```python
from build123d import *

# Parameters (mm, degrees)
BOSS_EXTRUDE1_DEPTH = 10
SKETCH2_R           = 11.75
BOSS_EXTRUDE2_DEPTH = 40
BOSS_EXTRUDE3_DEPTH = 20
CUT_EXTRUDE1_DEPTH  = 16
CUT_EXTRUDE2_DEPTH  = 10
CHAMFER1_SIZE       = 2
CHAMFER1_SIZE2      = 5.494954839


with BuildPart() as part:
    # Sketch1 → Boss-Extrude1 (new body)
    with BuildSketch(Plane(origin=(0, 0, 0), x_dir=(1, 0, 0), z_dir=(0, 1, 0))):
        Polygon((21.75, 12.557368355), (0, 25.11473671), (-21.75, 12.557368355), (-21.75, -12.557368355), (0, -25.11473671), (21.75, -12.557368355), align=None)
        Polygon((15.25, 8.804591605), (0, 17.60918321), (-15.25, 8.804591605), (-15.25, -8.804591605), (0, -17.60918321), (15.25, -8.804591605), align=None, mode=Mode.SUBTRACT)
    extrude(amount=BOSS_EXTRUDE1_DEPTH)

    # Sketch2 → Boss-Extrude2 (add)
    with BuildSketch(Plane.XZ):
        Polygon((21.75, 12.557368355), (0, 25.11473671), (-21.75, 12.557368355), (-21.75, -12.557368355), (0, -25.11473671), (21.75, -12.557368355), align=None)
        with Locations(Location((0, 0, 0), (0, 0, 270))):
            Circle(SKETCH2_R, mode=Mode.SUBTRACT)
    extrude(amount=BOSS_EXTRUDE2_DEPTH)

    # Sketch3 → Boss-Extrude3 (add)
    with BuildSketch(Plane.XZ.offset(40)):
        Polygon((21.75, 12.557368355), (0, 25.11473671), (-21.75, 12.557368355), (-21.75, -12.557368355), (0, -25.11473671), (21.75, -12.557368355), align=None)
    extrude(amount=BOSS_EXTRUDE3_DEPTH)

    # Sketch4 → Cut-Extrude1 (cut)
    with BuildSketch(Plane.XZ.offset(60)):
        with BuildLine():
            Line((-2.618090908, 1.66), (-2.618090908, -1.66))
            ThreePointArc((-2.618090908, -1.66), (3.1, 0), (-2.618090908, 1.66))
        make_face()
    extrude(amount=-CUT_EXTRUDE1_DEPTH, mode=Mode.SUBTRACT)

    # Sketch5 → Cut-Extrude2 (cut)
    with BuildSketch(Plane(origin=(0, 10, 0), x_dir=(1, 0, 0), z_dir=(0, 1, 0))):
        Polygon((8.804591605, 15.25), (-8.804591605, 15.25), (-17.60918321, 0), (-8.804591605, -15.25), (8.804591605, -15.25), (17.60918321, 0), align=None)
    extrude(amount=-CUT_EXTRUDE2_DEPTH, mode=Mode.SUBTRACT)

    # Chamfer1
    chamfer1_edges = [part.edges().sort_by_distance(p)[0] for p in [
        (-13.206887408, 10, -9.98418321),
        (2.043112592, 10, -16.429591605),
        (15.25, 10, -6.445408395),
        (16.429591605, 10, 2.043112592),
        (16.429591605, 10, -2.043112592),
        (9.98418321, 10, -13.206887408),
        (6.445408395, 10, -15.25),
        (-6.445408395, 10, -15.25),
        (-9.98418321, 10, -13.206887408),
        (-16.429591605, 10, -2.043112592),
        (-16.429591605, 10, 2.043112592),
        (-9.98418321, 10, 13.206887408),
        (-6.445408395, 10, 15.25),
        (6.445408395, 10, 15.25),
        (9.98418321, 10, 13.206887408),
        (15.25, 10, 6.445408395),
        (13.206887408, 10, -9.98418321),
        (-2.043112592, 10, -16.429591605),
        (-15.25, 10, -6.445408395),
        (-13.206887408, 10, 9.98418321),
        (2.043112592, 10, 16.429591605),
        (13.206887408, 10, 9.98418321),
        (-2.043112592, 10, 16.429591605),
        (-15.25, 10, 6.445408395),
    ]]
    chamfer1_side = [part.faces().sort_by_distance(p)[0] for p in [
        (10.542763262, 10, -18.260601622),
    ]]
    chamfer(chamfer1_edges, length=CHAMFER1_SIZE, length2=CHAMFER1_SIZE2, reference=chamfer1_side[0])


solid = part.part
```
Model file for the job. Use its own axes, mm. A direction names the side the tool comes from. Coordinates: 2 decimals unless noted, no trailing zeros. Order: outer loops, then holes, each group sorted by start corner. A loop starts at its lowest first (then second) coordinate and runs counter-clockwise, first axis right, second up. Notation, with made-up numbers: (-6.75, 58) -> (46.25, 58) arc R26 ccw to (46.25, 75) -> close; hole circle Ø8 at (-29, -38.5). An arc over 180 degrees is marked (long way). Return JSON: item names as keys, results as strings.
Item 1: Slice it at A-A (y = -32). Write the cut outline in (x, z).
Model answer:
{"outline": "(-21.75, -12.56) -> (0, -25.11) -> (21.75, -12.56) -> (21.75, 12.56) -> (0, 25.11) -> (-21.75, 12.56) -> close; hole circle Ø23.5 at (0, 0)"}
Item 2: Slice it at D-D (x = -6.5). Write the cut outline in (y, z), then the cut area to 3 significant figures.
Model answer:
{"outline": "(-60, -21.36) -> (10, -21.36) -> (10, -17.25) -> (4.51, -15.25) -> (0, -15.25) -> (0, -9.79) -> (-40, -9.79) -> (-40, 9.79) -> (0, 9.79) -> (0, 15.25) -> (4.51, 15.25) -> (10, 17.25) -> (10, 21.36) -> (-60, 21.36) -> close", "area": "1,890 mm²"}
Item 3: Slice it at B-B (z = -7.5). Write the cut outline in (x, y), then the cut area to 3 significant figures.
Model answer:
{"outline": "(-21.75, -60) -> (21.75, -60) -> (21.75, 10) -> (17.25, 10) -> (15.25, 4.51) -> (15.25, 0) -> (9.05, 0) -> (9.05, -40) -> (-9.05, -40) -> (-9.05, 0) -> (-15.25, 0) -> (-15.25, 4.51) -> (-17.25, 10) -> (-21.75, 10) -> close", "area": "2,010 mm²"}
Item 4: Pin check, flat tips, straight feed: P1, Ø10, axis at x = 0, z = 0, coming from the +Y side; P2, Ø8, axis at y = -12.5, z = -19.5, coming from the +X side; P3, Ø1.5, axis at x = 10, z = 10.5, coming from the +Y side. Stop position of each tip, or through.
Model answer:
{"P1": "stops at y = -40", "P2": "stops at x = 16.65", "P3": "stops at y = 0"}
Item 5: Slice it at C-C (y = -51.5). Write the cut outline in (x, z), then the cut area to 3 significant figures.
Model answer:
{"outline": "(-21.75, -12.56) -> (0, -25.11) -> (21.75, -12.56) -> (21.75, 12.56) -> (0, 25.11) -> (-21.75, 12.56) -> close; hole (-2.62, -1.66) arc R3.1 ccw (long way) to (-2.62, 1.66) -> close", "area": "1,610 mm²"}
Item 6: 3-axis set-ups, long thin cutter, end or side, ignore diameter. For faces 1 (the face through (-13.235, 2.221, 9.968)), 2 (the face through (3.1, -52.1, -0.1)): which of +Z, -Z, +X, -X, +Y, -Y reach the whole face in a straight line?
Model answer:
{"face 1": "+Y", "face 2": "-Y"}
Item 7: Wall check: line 1 along X through (y, z) = (-21, 0); line 2 along Z through (x, y) = (0, -48); line 3 along Y through (x, z) = (9, 5). Give the ranges that are in metal, low to high. Write a range as from..to.
Model answer:
{"line 1": "x = -21.75..-11.75, 11.75..21.75", "line 2": "z = -25.11..-3.1, 3.1..25.11", "line 3": "y = -60..-40"}
